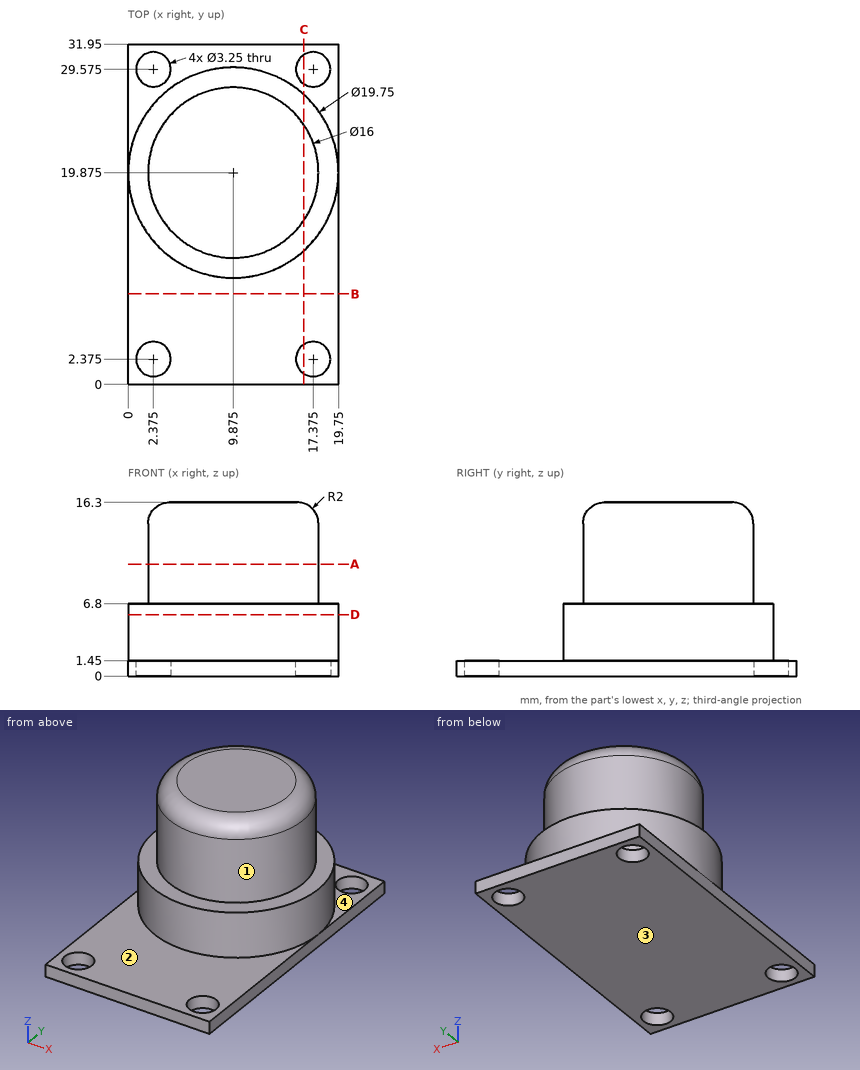
Design review of the part shown in the three views and the two pictorial views. Dimensions are in mm from the part's minimum x, y and z. A direction names the side the tool comes from. Coordinates: 2 decimals unless noted, no trailing zeros. Order: outer loops, then holes, each group sorted by start corner. A loop starts at its lowest first (then second) coordinate and runs counter-clockwise, first axis right, second up.
Item 1: Take a section at A-A, the plane z = 10.5. Write out the cut boundary in (x, y) (3 decimals).
Item 2: For line 1 (Z direction, x = 4.25, y = 29.5); line 2 (Z direction, x = 1.5, y = 18.5); line 3 (Y direction, x = 16, z = 11), list the stretches that pass through material, from the lowest coordinate up.
Item 3: For pin 1 Ø3.5 at (x, y) = (6, 27.5) entering from +Z; pin 2 Ø1 at (y, z) = (26, 5) entering from +X; pin 3 Ø5 at (x, y) = (2.375, 2.375) entering from +Z, all flat-tipped, find the tip position at first contact; note any pin that passes through.
Item 4: Take a section at C-C, the plane x = 16.5. Count the separate pieces of the cut face and the enclosed holes in it, then the cut area to 3 significant figures.
Item 5: Take a section at D-D, the plane z = 5.75. Write out the cut boundary in (x, y) (3 decimals).
Item 6: Take a section at B-B, the plane y = 8.5. Write out the cut boundary in (x, z).
Item 7: For the marked faces 1, 2, 3 and 4, list the 3-axis set-ups (+Z, -Z, +X, -X, +Y, -Y) from which the entire face can be reached by the end or side of a thin tool; tool diameter is ignored.
The answers:
1. outline: circle Ø16 at (9.875, 19.875)
2. line 1: z = 0 to 1.45
2. line 2: z = 0 to 6.8
2. line 3: y = 14.73 to 25.02
3. pin 1: stops at z = 16.13
3. pin 2: stops at x = 17.99
3. pin 3: stops at z = 1.45
4. separate pieces: 3
4. enclosed holes: 0
4. area: 198 mm2
5. outline: circle Ø19.75 at (9.875, 19.875)
6. outline: (0, 0) - (19.75, 0) - (19.75, 1.45) - (0, 1.45) - close
7. face 1: +Z
7. face 2: +Z, -Y
7. face 3: -Z, +X, -X, +Y, -Y
7. face 4: +Z, +Y
